Work out the finished part from the listing and answer in its coordinate system (mm). Round coordinates to 2 decimals unless told otherwise and drop trailing zeros. Return JSON: item names as keys, results as strings.
Autodesk Inventor part; units mm, degrees
ref_plane "YZ Plane" through (0, 0, 0) normal (1, 0, 0) x (0, 1, 0)
ref_plane "XZ Plane" through (0, 0, 0) normal (0, 1, 0) x (-1, 0, 0)
ref_plane "XY Plane" through (0, 0, 0) normal (0, 0, 1) x (1, 0, 0)
ref_plane "Work Plane1" through (-138.8109, 23.0767, 114.3) normal (0, 0, 1) x (1, 0, 0)
sketch "Sketch1" plane through (-138.8109, 23.0767, 114.3) normal (0, 0, 1) x (1, 0, 0)
  spline S0 degree 4 poles (0, 95.25) (-76.2, 95.25) (-95.25, 95.25) (-95.25, 76.2) (-95.25, 0) knots 1 1 1 1 1 2 2 2 2 2
  spline S1 degree 4 poles (95.25, 0) (95.25, 76.2) (95.25, 95.25) (76.2, 95.25) (0, 95.25) knots 1 1 1 1 1 2 2 2 2 2
  spline S2 degree 4 poles (0, -95.25) (76.2, -95.25) (95.25, -95.25) (95.25, -76.2) (95.25, 0) knots 1 1 1 1 1 2 2 2 2 2
  spline S3 degree 4 poles (-95.25, 0) (-95.25, -76.2) (-95.25, -95.25) (-76.2, -95.25) (0, -95.25) knots 1 1 1 1 1 2 2 2 2 2
  line L0 (0, 95.25) -> (0, -95.25) construction
  line L1 (95.25, 0) -> (-95.25, 0) construction
  spline S4 degree 3 poles (-93.6625, 0) (-93.6625, 13.1515) (-93.6641, 24.3836) (-93.4921, 34.0057) (-93.1277, 54.3921) (-91.9513, 67.5764) (-88.2745, 76.0527) (-86.2377, 80.7481) (-83.4985, 84.0104) (-79.5283, 86.4707) (-74.4505, 89.6173) (-67.2348, 91.4109) (-56.937, 92.4035) (-43.6826, 93.6811) (-25.4087, 93.6625) (0, 93.6625) knots -2 -2 -2 -2 -1.870556 -1.870556 -1.870556 -1.596305 -1.596305 -1.596305 -1.444385 -1.444385 -1.444385 -1.250085 -1.250085 -1.250085 -1 -1 -1 -1 construction
  spline S5 degree 3 poles (0, 93.6625) (13.1515, 93.6625) (24.3836, 93.6642) (34.0057, 93.4922) (54.392, 93.1278) (67.5764, 91.9513) (76.0526, 88.2745) (80.748, 86.2378) (84.0104, 83.4986) (86.4706, 79.5283) (89.6173, 74.4505) (91.4109, 67.2348) (92.4035, 56.937) (93.681, 43.6826) (93.6625, 25.4087) (93.6625, 0) knots -2 -2 -2 -2 -1.870556 -1.870556 -1.870556 -1.596305 -1.596305 -1.596305 -1.444385 -1.444385 -1.444385 -1.250085 -1.250085 -1.250085 -1 -1 -1 -1 construction
  spline S6 degree 3 poles (0, -93.6625) (-13.1515, -93.6625) (-24.3836, -93.6641) (-34.0057, -93.4921) (-54.392, -93.1277) (-67.5764, -91.9512) (-76.0526, -88.2744) (-80.748, -86.2377) (-84.0104, -83.4985) (-86.4706, -79.5283) (-89.6173, -74.4505) (-91.4109, -67.2347) (-92.4035, -56.9369) (-93.681, -43.6826) (-93.6625, -25.4086) (-93.6625, 0) knots -2 -2 -2 -2 -1.870556 -1.870556 -1.870556 -1.596305 -1.596305 -1.596305 -1.444385 -1.444385 -1.444385 -1.250085 -1.250085 -1.250085 -1 -1 -1 -1 construction
  spline S7 degree 3 poles (93.6625, 0) (93.6625, -13.1514) (93.6641, -24.3836) (93.4921, -34.0057) (93.1277, -54.392) (91.9513, -67.5763) (88.2745, -76.0526) (86.2377, -80.748) (83.4985, -84.0103) (79.5283, -86.4706) (74.4505, -89.6172) (67.2348, -91.4108) (56.937, -92.4034) (43.6826, -93.681) (25.4087, -93.6625) (0, -93.6625) knots -2 -2 -2 -2 -1.870556 -1.870556 -1.870556 -1.596305 -1.596305 -1.596305 -1.444385 -1.444385 -1.444385 -1.250085 -1.250085 -1.250085 -1 -1 -1 -1 construction
  line L2 (-63.5, 63.5) -> (63.5, 63.5) construction
  line L3 (63.5, 63.5) -> (63.5, -63.5) construction
  line L4 (63.5, -63.5) -> (-63.5, -63.5) construction
  line L5 (-63.5, -63.5) -> (-63.5, 63.5) construction
  circle A0 centre (0, 0) radius 85.725
  circle A1 centre (63.5, 63.5) radius 3.175
  circle A2 centre (-63.5, 63.5) radius 3.175
  circle A3 centre (-63.5, -63.5) radius 3.175
  circle A4 centre (63.5, -63.5) radius 3.175
  point P0 (138.8109, -23.0767)
  dimension "d0" = 127
  dimension "d1" = 127
  dimension "d2" = 63.5
  dimension "d3" = 63.5
  dimension "d4" = 171.45
  dimension "d7" = 6.35
  dimension "d8" = 6.35
  dimension "d9" = 6.35
  dimension "d10" = 6.35
extrude "Extrusion1" add sketch "Sketch1" along normal blind 2.75
properties part number "Frame Lower"
Item 1: Consider line 1 along Y through (x, z) = (-202, 114.8); line 2 along Y through (x, z) = (-76, 116.15); line 3 along X through (y, z) = (-10, 115.8). Determine where each line is inside the solid, lowest interval first. Write a range as [from, to].
Output:
{"line 1": "y = [-70.17, -43.58], [-37.26, -34.85], [81.01, 83.42], [89.74, 116.33]", "line 2": "y = [-70.23, -43.52], [-37.32, -35.26], [81.42, 83.48], [89.68, 116.38]", "line 3": "x = [-233.91, -217.9], [-59.72, -43.72]"}
Item 2: Find section A-A (z = 116.1). State how many separate pieces and enclosed holes the cut face has, plus the area to 3 significant figures.
Output:
{"separate pieces": "1", "enclosed holes": "5", "area": "11,600 mm^2"}
Item 3: The mould has two halves that part along Y. Classify faces 1 (the flat face through (-175, 101, 114.3)), 2 (the cylindrical face through (-78.483, -40.563, 115.656)): pulls with the +Y half, pulls with the -Y half, needs draft (parallel to the pull), parting line crosses it, or undercut.
Output:
{"face 1": "needs draft", "face 2": "undercut"}
